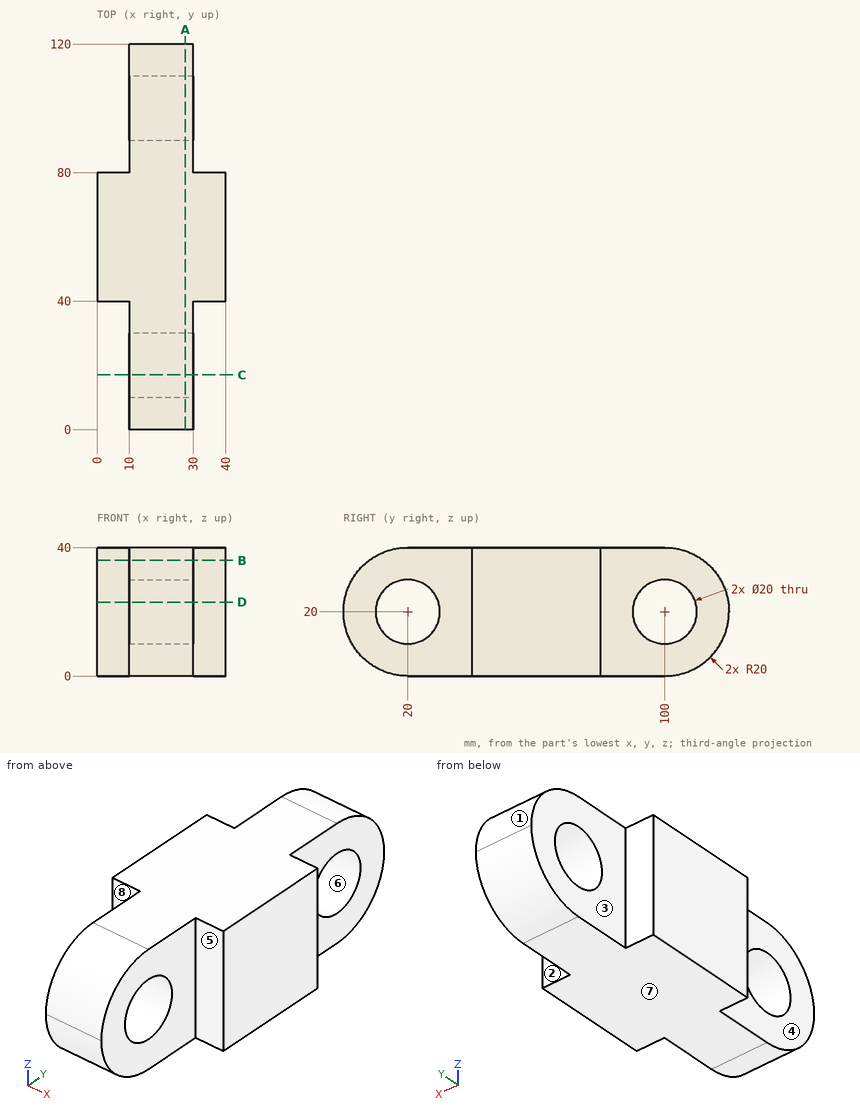
Could you check a few things on this drawing? It's one solid part, dimensions in mm from its lowest x, y, z. A direction names the side the tool comes from. Coordinates: 2 decimals unless noted, no trailing zeros. Write each loop counter-clockwise with the first axis right and the second up, starting at its lowest first coordinate (ties: lowest second). Pieces come first, ordered by that corner, then holes.
Q1. Imagine slicing it at D-D, the plane z = 23. List the corners of the cut face in (x, y) for me, plus the area to 3 significant figures.
Results found:
outline: (0, 40) - (10, 40) - (10, 29.54) - (30, 29.54) - (30, 40) - (40, 40) - (40, 80) - (30, 80) - (30, 90.46) - (10, 90.46) - (10, 80) - (0, 80) - close; (10, 0.23) - (30, 0.23) - (30, 10.46) - (10, 10.46) - close; (10, 109.54) - (30, 109.54) - (30, 119.77) - (10, 119.77) - close
area: 2,430 mm2
Q2. Imagine slicing it at B-B, the plane z = 36. List the corners of the cut face in (x, y) for me.
Results found:
outline: (0, 40) - (10, 40) - (10, 8) - (30, 8) - (30, 40) - (40, 40) - (40, 80) - (30, 80) - (30, 112) - (10, 112) - (10, 80) - (0, 80) - close
Q3. Imagine slicing it at A-A, the plane x = 27.5. Count the separate pieces of the cut face and the enclosed holes in it, plus the area to 3 significant figures.
Results found:
separate pieces: 1
enclosed holes: 2
area: 3,830 mm2
Q4. Please list where these lines run through material, in increasing order: L1, parallel to Y at x = 13.5, z = 15; L2, parallel to Y at x = 15, z = 24; L3, parallel to Z at x = 15, y = 100.
Results found:
L1: y = 0.64 to 11.34, 28.66 to 91.34, 108.66 to 119.36
L2: y = 0.4 to 10.83, 29.17 to 90.83, 109.17 to 119.6
L3: z = 0 to 10, 30 to 40
Q5. If we mould it in two halves opening along Z, with no side actions, what happens to the marked faces 6, 7 and 8? For each: +Z half, -Z half, draft (parallel to the pull), parting line (faces both ways), or undercut.
Results found:
face 6: undercut
face 7: -Z half
face 8: draft
Q6. Which directions (+Z, -Z, +X, -X, +Y, -Y) give clear straight access to the entire face, cutting with the end or side of a thin tool? Please do the marked faces 1, 2, 3, 4 and 5.
Results found:
face 1: +Z, +X, -X, +Y
face 2: +Z, -Z, +X, +Y
face 3: +Z, -Z, -X, +Y
face 4: +Z, -Z, -X, -Y
face 5: +Z, -Z, +X, -Y
Q7. For P1, Ø3, axis at x = 13, z = 4.5, coming from the -Y side; P2, Ø11, axis at x = 37, z = 25.5, coming from the +Y side; P3, Ø4, axis at x = 21, z = 4, coming from the +Y side, each with a flat end and sliding along its axis, tell me the tip position at first contact or that it passes through.
Results found:
P1: stops at y = 5.72
P2: stops at y = 80
P3: stops at y = 114.28
Q8. Imagine slicing it at C-C, the plane y = 17. List the corners of the cut face in (x, z) for me, plus the area to 3 significant figures.
Results found:
outline: (10, 0.23) - (30, 0.23) - (30, 10.46) - (10, 10.46) - close; (10, 29.54) - (30, 29.54) - (30, 39.77) - (10, 39.77) - close
area: 409 mm2
